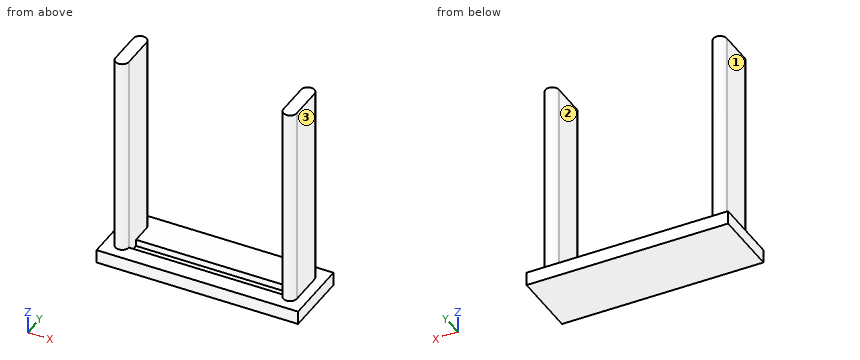
from build123d import *

# Parameters (mm, degrees)
CROQUIS1_W              = 30
CROQUIS1_H              = 10
SALIENTE_EXTRUIR1_DEPTH = 2
SALIENTE_EXTRUIR2_DEPTH = 20
CROQUIS3_W              = 23
CROQUIS3_H              = 2
CORTAR_EXTRUIR1_DEPTH   = 1
SALIENTE_EXTRUIR3_DEPTH = 10


with BuildPart() as part:
    # Croquis1 → Saliente-Extruir1 (new body)
    with BuildSketch(Plane.XY):
        Rectangle(CROQUIS1_W, CROQUIS1_H)
    extrude(amount=SALIENTE_EXTRUIR1_DEPTH)

    # Croquis2 → Saliente-Extruir2 (add)
    with BuildSketch(Plane.XY.offset(2)):
        with BuildLine():
            Line((-13.5, -2.5), (-13.5, 2.5))
            ThreePointArc((-13.5, 2.5), (-12.5, 3.5), (-11.5, 2.5))
            Line((-11.5, 2.5), (-11.5, -2.5))
            ThreePointArc((-11.5, -2.5), (-12.5, -3.5), (-13.5, -2.5))
        make_face()
        with BuildLine():
            Line((11.5, 2.5), (11.5, -2.5))
            ThreePointArc((11.5, -2.5), (12.5, -3.5), (13.5, -2.5))
            Line((13.5, -2.5), (13.5, 2.5))
            ThreePointArc((13.5, 2.5), (12.5, 3.5), (11.5, 2.5))
        make_face()
    extrude(amount=SALIENTE_EXTRUIR2_DEPTH)

    # Croquis3 → Cortar-Extruir1 (cut)
    with BuildSketch(Plane.XY.offset(2)):
        with Locations((0, -1.5)):
            Rectangle(CROQUIS3_W, CROQUIS3_H)
    extrude(amount=-CORTAR_EXTRUIR1_DEPTH, mode=Mode.SUBTRACT)

    # Croquis4 → Saliente-Extruir3 (add)
    with BuildSketch(Plane.XY.offset(22)):
        with BuildLine():
            Line((-13.5, 2.5), (-11.5, 2.5))
            ThreePointArc((-11.5, 2.5), (-12.5, 3.5), (-13.5, 2.5))
        make_face()
        with BuildLine():
            ThreePointArc((-11.5, 2.5), (-12.5, 3.5), (-13.5, 2.5))
            Line((-13.5, 2.5), (-11.5, 2.5))
        make_face()
        with BuildLine():
            Line((-11.5, 2.5), (-13.5, 2.5))
            ThreePointArc((-13.5, 2.5), (-12.5, 1.5), (-11.5, 2.5))
        make_face()
        with BuildLine():
            ThreePointArc((-11.5, 2.5), (-12.5, 1.5), (-13.5, 2.5))
            Line((-13.5, 2.5), (-13.5, -2.5))
            ThreePointArc((-13.5, -2.5), (-12.5, -1.5), (-11.5, -2.5))
            Line((-11.5, -2.5), (-11.5, 2.5))
        make_face()
        with BuildLine():
            Line((-13.5, -2.5), (-11.5, -2.5))
            ThreePointArc((-11.5, -2.5), (-12.5, -3.5), (-13.5, -2.5))
        make_face()
        with BuildLine():
            ThreePointArc((-11.5, -2.5), (-12.5, -1.5), (-13.5, -2.5))
            Line((-13.5, -2.5), (-11.5, -2.5))
        make_face()
        with BuildLine():
            Line((-11.5, -2.5), (-13.5, -2.5))
            ThreePointArc((-13.5, -2.5), (-12.5, -3.5), (-11.5, -2.5))
        make_face()
        with BuildLine():
            ThreePointArc((13.5, -2.5), (12.5, -1.5), (11.5, -2.5))
            Line((11.5, -2.5), (13.5, -2.5))
        make_face()
        with BuildLine():
            Line((13.5, -2.5), (11.5, -2.5))
            ThreePointArc((11.5, -2.5), (12.5, -3.5), (13.5, -2.5))
        make_face()
        with BuildLine():
            ThreePointArc((13.5, 2.5), (12.5, 1.5), (11.5, 2.5))
            Line((11.5, 2.5), (11.5, -2.5))
            ThreePointArc((11.5, -2.5), (12.5, -1.5), (13.5, -2.5))
            Line((13.5, -2.5), (13.5, 2.5))
        make_face()
        with BuildLine():
            ThreePointArc((13.5, 2.5), (12.5, 3.5), (11.5, 2.5))
            Line((11.5, 2.5), (13.5, 2.5))
        make_face()
        with BuildLine():
            Line((13.5, 2.5), (11.5, 2.5))
            ThreePointArc((11.5, 2.5), (12.5, 1.5), (13.5, 2.5))
        make_face()
    extrude(amount=SALIENTE_EXTRUIR3_DEPTH)


solid = part.part
Design review of the part built by this model. Coordinates are the model's own, in mm. Face numbers are marked on the shaded views. Give positions to 0.01 mm unless a question says otherwise; leave off trailing zeros. Loops run counter-clockwise (first coordinate to the right, second up) from the corner with the lowest first, then second, coordinate; pieces in that order, holes last. Notation, with made-up numbers: M 50,7 L 66,7 A25 cw 66,31 Z; hole C 20.25,54.25 d5. An arc over 180 degrees is marked long. Answer as a JSON object with one key per item and string values.
Item 1: For P1, Ø5, axis at y = 1, z = 6, coming from the -X side; P2, Ø4, axis at y = -0.5, z = 9.5, coming from the +X side; P3, Ø4, axis at x = -11.5, y = 1, coming from the -Z side; P4, Ø3, axis at x = 0, y = 0, coming from the +Z side, all flat-tipped, find the tip position at first contact; note any pin that passes through.
Output values:
{"P1": "stops at x = -13.5", "P2": "stops at x = 13.5", "P3": "stops at z = 0", "P4": "stops at z = 2"}
Item 2: We need section D-D (x = -12.5). State the section outline as (y, z) points.
Output values:
{"outline": "M -5,0 L 5,0 L 5,2 L 3.5,2 L 3.5,32 L -3.5,32 L -3.5,2 L -5,2 Z"}
Item 3: Wall thickness on line 1 along X through (y, z) = (1, 22.5); line 2 along Z through (x, y) = (10.25, -4); line 3 along Z through (x, y) = (-6.5, -1.5): over which ranges is each line inside the solid? List them lowest first.
Output values:
{"line 1": "x = -13.5 to -11.5, 11.5 to 13.5", "line 2": "z = 0 to 2", "line 3": "z = 0 to 1"}
Item 4: We need section B-B (x = -2.5). State the section outline as (y, z) points.
Output values:
{"outline": "M -5,0 L 5,0 L 5,2 L -0.5,2 L -0.5,1 L -2.5,1 L -2.5,2 L -5,2 Z"}
Item 5: Mouldability with a two-part tool opening along X and no side actions: class the marked faces 1, 2 and 3 as pulls with the +X half, pulls with the -X half, needs draft (parallel to the pull), parting line crosses it, or undercut.
Output values:
{"face 1": "pulls with the -X half", "face 2": "undercut", "face 3": "pulls with the +X half"}
Item 6: We need section C-C (y = 0). State the section outline as (x, z) points, and give its area (3 significant figures).
Output values:
{"outline": "M -15,0 L 15,0 L 15,2 L 13.5,2 L 13.5,32 L 11.5,32 L 11.5,2 L -11.5,2 L -11.5,32 L -13.5,32 L -13.5,2 L -15,2 Z", "area": "180 mm2"}
Item 7: We need section A-A (z = 28). State the section outline as (x, y) points.
Output values:
{"outline": "M -13.5,-2.5 A1 ccw -11.5,-2.5 L -11.5,2.5 A1 ccw -13.5,2.5 Z; M 11.5,-2.5 A1 ccw 13.5,-2.5 L 13.5,2.5 A1 ccw 11.5,2.5 Z"}
